Input: dimensioned drawing with shaded views. Units: mm. Origin: part minimum x, y, z. Give positions to 0.01 mm unless a question says otherwise; leave off trailing zeros. Loops run counter-clockwise (first coordinate to the right, second up) from the corner with the lowest first, then second, coordinate; pieces in that order, holes last.
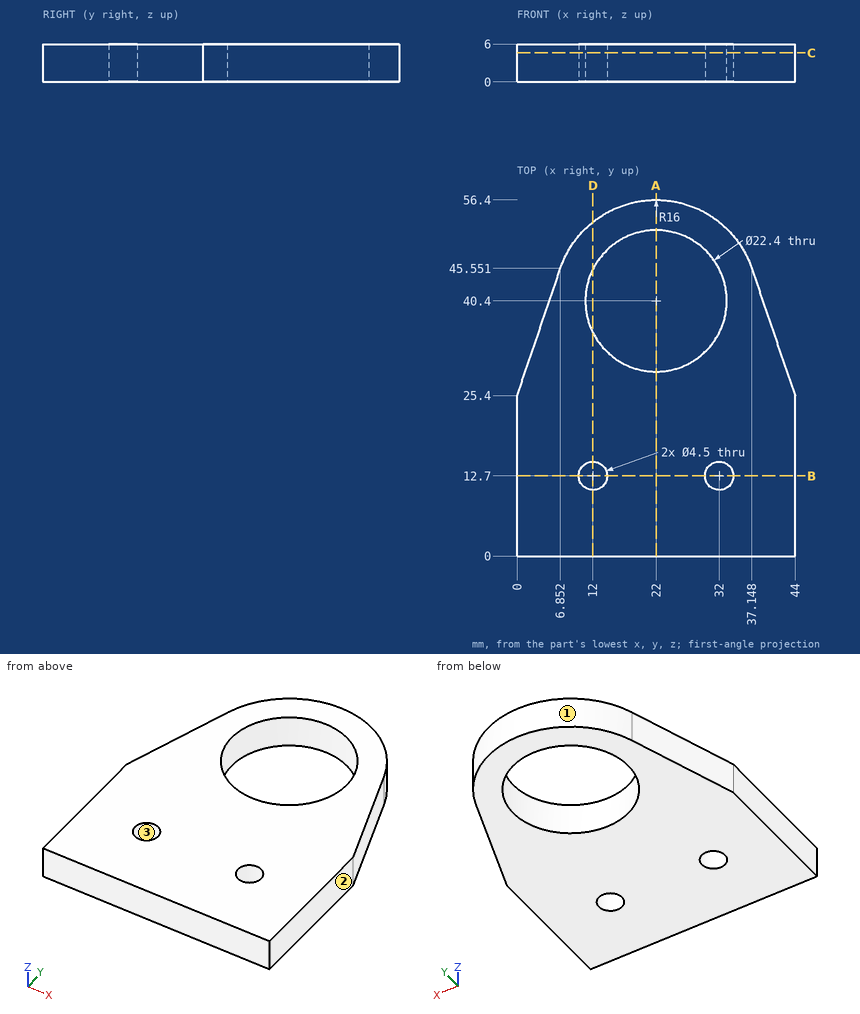
(1) Mould query, pull axis X, two halves, no side actions, for the marked faces 1, 2 and 3. Classes: pulls with the +X half, pulls with the -X half, needs draft (parallel to the pull), parting line crosses it, or undercut.
A:
face 1: parting line crosses it
face 2: pulls with the +X half
face 3: undercut
(2) Section A-A, the plane x = 22. Return the cut outline in (y, z).
A:
outline: (0, 0) - (29.2, 0) - (29.2, 6) - (0, 6) - close; (51.6, 0) - (56.4, 0) - (56.4, 6) - (51.6, 6) - close
(3) First-contact query: pin 1 (18 mm diameter, centred on x = 22, y = 40.4, fed in from +Z); pin 2 (2 mm diameter, centred on x = 9, z = 4, fed in from +Y). Flat tips, straight axial feed; report the tip coordinate or a pass-through.
A:
pin 1: passes through
pin 2: stops at y = 50.98
(4) Ray query, line 1 along Y through (x, z) = (22, 3.7); line 2 along X through (y, z) = (44, 5.65) (1 decimal); line 3 along X through (y, z) = (34.5, 2.05) (1 decimal). Return the intervals inside material, ascending.
A:
line 1: y = 0 to 29.2, 51.6 to 56.4
line 2: x = 6.3 to 11.4, 32.6 to 37.7
line 3: x = 3.1 to 12.5, 31.5 to 40.9
(5) Section B-B, the plane y = 12.7. Return the cut outline in (x, z).
A:
outline: (0, 0) - (9.75, 0) - (9.75, 6) - (0, 6) - close; (14.25, 0) - (29.75, 0) - (29.75, 6) - (14.25, 6) - close; (34.25, 0) - (44, 0) - (44, 6) - (34.25, 6) - close
(6) Section C-C, the plane z = 4.6. Return the cut outline in (x, y).
A:
outline: (0, 0) - (44, 0) - (44, 25.4) - (37.15, 45.55) arc R16 ccw to (6.85, 45.55) - (0, 25.4) - close; hole circle Ø4.5 at (12, 12.7); hole circle Ø22.4 at (22, 40.4); hole circle Ø4.5 at (32, 12.7)
(7) Section D-D, the plane x = 12. Return the cut outline in (y, z).
A:
outline: (0, 0) - (10.45, 0) - (10.45, 6) - (0, 6) - close; (14.95, 0) - (35.36, 0) - (35.36, 6) - (14.95, 6) - close; (45.44, 0) - (52.89, 0) - (52.89, 6) - (45.44, 6) - close
